```python
from build123d import *

# Parameters (mm, degrees)
SKETCH1_W           = 21.5
SKETCH1_H           = 36
BOSS_EXTRUDE1_DEPTH = 1.5
SKETCH2_W           = 14.5
SKETCH2_H           = 1
BOSS_EXTRUDE2_DEPTH = 3


with BuildPart() as part:
    # Sketch1 → Boss-Extrude1 (new body)
    with BuildSketch(Plane.XY):
        with Locations((10.75, 18)):
            Rectangle(SKETCH1_W, SKETCH1_H)
    extrude(amount=BOSS_EXTRUDE1_DEPTH)

    # Sketch2 → Boss-Extrude2 (add)
    with BuildSketch(Plane.XY.offset(1.5)):
        Polygon((3.75, 0), (4.75, 0), (4.75, 1), (4.75, 30), (3.75, 30), align=None)
        with Locations((12, 0.5)):
            Rectangle(SKETCH2_W, SKETCH2_H)
        Polygon((19.25, 0), (20.25, 0), (20.25, 31), (19.25, 31), (19.25, 30), (19.25, 1), align=None)
        Polygon((19.25, 30), (19.25, 31), (3.75, 31), (3.75, 30), (4.75, 30), align=None)
    extrude(amount=-BOSS_EXTRUDE2_DEPTH)


solid = part.part
```
Here's how the part is built. I have some questions about the finished solid (model axes, mm). A direction names the side the tool comes from. Round coordinates to 2 decimals unless told otherwise and drop trailing zeros. Order: outer loops, then holes, each group sorted by start corner. A loop starts at its lowest first (then second) coordinate and runs counter-clockwise, first axis right, second up. Notation, with made-up numbers: (-33, 89.25) -> (14, 89.25) arc R35 ccw to (14, 123.25) -> close; hole circle Ø5 at (5, 57). An arc over 180 degrees is marked (long way). Use a Markdown table: item, result. Add a question column.
(1) If we mould it in two halves opening along Y, with no side actions, what happens to faces 6 (the face through (11, 0, 0)), 7 (the face through (12, 31, -1)), 8 (the face through (4.75, 15, -1)), 9 (the face through (3.5, 20.8, 0))? For each: released by +Y, released by -Y, zero draft, split by the parting line, or undercut.
(2) I need wall thicknesses on line 1 along X through (y, z) = (18.5, -0.7); line 2 along Y through (x, z) = (12.75, -1); line 3 along Z through (x, y) = (12.25, 32). Which ranges of each line are inside material? Lowest first, please.
(3) Suppose I cut it at A-A, the plane z = -1.05. Please give me the cut outline in (x, y), and give its area (3 significant figures).
(4) Suppose I cut it at D-D, the plane x = 4.25. Please give me the cut outline in (y, z), and give its area (4 significant figures).
(5) Suppose I cut it at B-B, the plane x = 8. Please give me the cut outline in (y, z), and give its area (3 significant figures).
(6) Suppose I cut it at C-C, the plane y = 8. Please give me the cut outline in (x, z), and give its area (4 significant figures).
(7) For pin 1 Ø1.6 at (y, z) = (14.5, -1) entering from +X; pin 2 Ø0.8 at (x, z) = (9, -0.5) entering from +Y; pin 3 Ø1.6 at (y, z) = (11, -1) entering from -X, each with a flat end and sliding along its axis, tell me the tip position at first contact or that it passes through.
(8) For faces 1 (the face through (21.5, 18, 1)), 2 (the face through (3.75, 16, -1)), 3 (the face through (11, 36, 1)), 4 (the face through (12, 1, -1)), 5 (the face through (20.25, 15, -1)), which set-ups out of +Z, -Z, +X, -X, +Y, -Y let a thin tool reach every point of the face, with its end or its side?
Verdict:
| question | item | result |
|---|---|---|
| 1 | face 6 | released by -Y |
| 1 | face 7 | released by +Y |
| 1 | face 8 | undercut |
| 1 | face 9 | zero draft |
| 2 | line 1 | 3.75 to 4.75, 19.25 to 20.25 |
| 2 | line 2 | 0 to 1, 30 to 31 |
| 2 | line 3 | 0 to 1.5 |
| 3 | outline | (3.75, 0) -> (20.25, 0) -> (20.25, 31) -> (3.75, 31) -> close; hole (4.75, 1) -> (19.25, 1) -> (19.25, 30) -> (4.75, 30) -> close |
| 3 | area | 91.0 mm2 |
| 4 | outline | (0, -1.5) -> (31, -1.5) -> (31, 0) -> (36, 0) -> (36, 1.5) -> (0, 1.5) -> close |
| 4 | area | 100.5 mm2 |
| 5 | outline | (0, -1.5) -> (1, -1.5) -> (1, 0) -> (30, 0) -> (30, -1.5) -> (31, -1.5) -> (31, 0) -> (36, 0) -> (36, 1.5) -> (0, 1.5) -> close |
| 5 | area | 57.0 mm2 |
| 6 | outline | (0, 0) -> (3.75, 0) -> (3.75, -1.5) -> (4.75, -1.5) -> (4.75, 0) -> (19.25, 0) -> (19.25, -1.5) -> (20.25, -1.5) -> (20.25, 0) -> (21.5, 0) -> (21.5, 1.5) -> (0, 1.5) -> close |
| 6 | area | 35.25 mm2 |
| 7 | pin 1 | x = 20.25 |
| 7 | pin 2 | y = 31 |
| 7 | pin 3 | x = 3.75 |
| 8 | face 1 | +Z, -Z, +X, +Y, -Y |
| 8 | face 2 | -Z, -X, +Y, -Y |
| 8 | face 3 | +Z, -Z, +X, -X, +Y |
| 8 | face 4 | -Z |
| 8 | face 5 | -Z, +X, +Y, -Y |
